```python
from build123d import *

# Parameters (mm, degrees)
F1_DEPTH     = 3.81
F2_R         = 2.032
F3_T3_ANGLE  = 90
F3_T6_ANGLE  = 90
F3_T9_DEPTH  = 16.51
F3_T12_DEPTH = 16.51


# Not quite as in the source:
# - a fillet or chamfer that OpenCascade refuses, or shapes differently, is made with other operations: its cross-section is extruded or revolved along the edge and cut away or added


with BuildPart() as f1:
    # F0 (on Top) → F1 (new body)
    with BuildSketch(Plane.XY):
        with BuildLine():
            Line((0, 36.1550717625), (0, 0))
            Line((0, 0), (50.8, 0))
            Line((50.8, 0), (50.8, 36.1550717625))
            Line((50.8, 36.1550717625), (45.72, 36.1550717625))
            Line((45.72, 36.1550717625), (45.72, 99.06))
            ThreePointArc((45.72, 99.06), (25.4, 119.38), (5.08, 99.06))
            Line((5.08, 99.06), (5.08, 36.1550717625))
            Line((5.08, 36.1550717625), (0, 36.1550717625))
        make_face()
        Polygon((21.5968196758, 48.7659722567), (5.08, 5.08), (5.08, 30.9497844428), (10.16, 30.9497844428), (10.16, 85.6342857143), (21.623824299, 55.3370357813), (18.1859140491, 55.3370357813), (18.1859140491, 48.7659722567), align=None, mode=Mode.SUBTRACT)
        Polygon((40.64, 5.08), (10.1879829027, 5.08), (25.4079982621, 45.3360045931), align=None, mode=Mode.SUBTRACT)
        Polygon((45.72, 30.9497844428), (45.72, 5.08), (29.1901726596, 48.7659722567), (32.5980894268, 48.7659722567), (32.5980894268, 55.3370357813), (29.1891943801, 55.3370357813), (40.64, 85.6237124205), (40.64, 30.9497844428), align=None, mode=Mode.SUBTRACT)
        Polygon((25.3920017379, 58.8039954069), (12.6709696314, 92.4238659741), (24.3276693245, 92.4238659741), (26.4725103977, 92.4238659741), (38.1030234, 92.4238659741), align=None, mode=Mode.SUBTRACT)
        with BuildLine():
            ThreePointArc((10.16, 99.06), (25.3630832236, 114.3000449305), (40.64, 99.1340130568))
            Line((40.64, 99.1340130568), (36.7868717318, 97.3090561919))
            Line((36.7868717318, 97.3090561919), (29.223334248, 97.3090561919))
            ThreePointArc((29.223334248, 97.3090561919), (25.4000898611, 104.8685646157), (21.5768454742, 97.3090561919))
            Line((21.5768454742, 97.3090561919), (13.8981392212, 97.3090561919))
            Line((13.8981392212, 97.3090561919), (10.16, 99.06))
        make_face(mode=Mode.SUBTRACT)
    extrude(amount=F1_DEPTH)

    # F2
    f2_edges = [f1.edges().sort_by_distance(p)[0] for p in [
        (45.72, 67.607536, 3.81),
        (50.8, 18.077536, 3.81),
        (48.26, 36.155072, 3.81),
        (2.54, 36.155072, 3.81),
        (0, 18.077536, 3.81),
    ]]
    fillet(f2_edges, radius=F2_R)

    # F3: fillet of radius 5.08 on 2 edges, made by hand


with BuildPart() as f3_tool1:
    # F3_s2 → F3_t3 (revolve)
    with BuildSketch(Plane.YZ.offset(5.08)):
        with BuildLine():
            ThreePointArc((34.1230717625, 3.81), (35.5599127419, 3.2148409794), (36.1550717625, 1.778))
            Line((36.1550717625, 1.778), (36.1550717625, 3.81))
            Line((36.1550717625, 3.81), (34.1230717625, 3.81))
        make_face()
    revolve(axis=Axis((5.08, 31.0750717625, 3.81), (0, 0, 1)), revolution_arc=F3_T3_ANGLE)


with BuildPart() as f3_tool4:
    # F3_s5 → F3_t6 (revolve)
    with BuildSketch(Plane.XZ.offset(-31.0750717625)):
        with BuildLine():
            ThreePointArc((48.768, 3.81), (50.2048409794, 3.2148409794), (50.8, 1.778))
            Line((50.8, 1.778), (50.8, 3.81))
            Line((50.8, 3.81), (48.768, 3.81))
        make_face()
    revolve(axis=Axis((45.72, 31.0750717625, 3.81), (0, 0, 1)), revolution_arc=F3_T6_ANGLE)


with BuildPart() as f3_tool7:
    # F3_s8 → F3_t9 (new body)
    with BuildSketch(Plane.XY.offset(-12.7)):
        with BuildLine():
            ThreePointArc((50.8, 31.0750717625), (49.3121024484, 34.667174211), (45.72, 36.1550717625))
            Line((45.72, 36.1550717625), (50.8, 36.1550717625))
            Line((50.8, 36.1550717625), (50.8, 31.0750717625))
        make_face()
    extrude(amount=F3_T9_DEPTH)


with BuildPart() as f3_tool10:
    # F3_s11 → F3_t12 (new body)
    with BuildSketch(Plane.XY.offset(-12.7)):
        with BuildLine():
            ThreePointArc((5.08, 36.1550717625), (1.4878975516, 34.667174211), (0, 31.0750717625))
            Line((0, 31.0750717625), (0, 36.1550717625))
            Line((0, 36.1550717625), (5.08, 36.1550717625))
        make_face()
    extrude(amount=F3_T12_DEPTH)


with BuildPart() as f1_1:
    add(f1.part)

    # F3_t13: cut F3_tool1, F3_tool4, F3_tool7, F3_tool10
    add([f3_tool1.part, f3_tool4.part, f3_tool7.part, f3_tool10.part], mode=Mode.SUBTRACT)


solid = f1_1.part
```
Model file for the job. Use its own axes, mm. A direction names the side the tool comes from. Coordinates: 2 decimals unless noted, no trailing zeros. Order: outer loops, then holes, each group sorted by start corner. A loop starts at its lowest first (then second) coordinate and runs counter-clockwise, first axis right, second up. Notation, with made-up numbers: (24.5, 79) -> (71.5, 79) arc R36 cw to (71.5, 116) -> close; hole circle Ø6 at (30, 28.5). An arc over 180 degrees is marked (long way). Return JSON: item names as keys, results as strings.
Item 1: Slice it at B-B (z = 0.95). Count the separate pieces of the cut face and the enclosed holes in it, then the cut area to 3 significant figures.
Model answer:
{"separate pieces": "1", "enclosed holes": "5", "area": "2,650 mm²"}
Item 2: Wall check: line 1 along X through (y, z) = (21, 2.75); line 2 along X through (y, z) = (104, 3.35); line 3 along X through (y, z) = (69, 3.6). Give the ranges that are in metal, low to high. Write a range as from..to.
Model answer:
{"line 1": "x = 0.25..5.08, 11.1..16.21, 34.62..39.7, 45.72..50.55", "line 2": "x = 6.46..10.98, 22.66..28.14, 39.82..44.34", "line 3": "x = 6.21..10.16, 16.45..21.53, 29.25..34.35, 40.64..44.59"}
Item 3: 3-axis set-ups, long thin cutter, end or side, ignore diameter. For faces 1 (the face through (25, 0, 2)), 2 (the face through (31.836, 75.849, 1.878)): which of +Z, -Z, +X, -X, +Y, -Y reach the whole face in a straight line?
Model answer:
{"face 1": "+Z, -Z, +X, -X, -Y", "face 2": "+Z, -Z"}
Item 4: Pin check, flat tips, straight feed: P1, Ø2, axis at x = 7, y = 26.5, coming from the +Z side; P2, Ø1.9, axis at y = 53, z = 2.5, coming from the -X side; P3, Ø1, axis at y = 53.5, z = 2, coming from the +X side. Stop position of each tip, or through.
Model answer:
{"P1": "passes through", "P2": "stops at x = 5.08", "P3": "stops at x = 45.72"}
Item 5: Mould opens along X. For faces 3 (the face through (18, 97.309, 2)), 4 (the face through (15.81, 70.7, 1.88)), 5 (the face through (5.66, 66.14, 3.2)), 6 (the face through (50.22, 15.76, 3.2)) say: pulls with the +X half, pulls with the -X half, needs draft (parallel to the pull), parting line crosses it, or undercut.
Model answer:
{"face 3": "undercut", "face 4": "undercut", "face 5": "pulls with the -X half", "face 6": "pulls with the +X half"}
Item 6: Slice it at A-A (y = 13). Write the cut outline in (x, z).
Model answer:
{"outline": "(0, 0) -> (5.08, 0) -> (5.08, 3.81) -> (2.03, 3.81) arc R2.03 ccw to (0, 1.78) -> close; (8.07, 0) -> (13.18, 0) -> (13.18, 3.81) -> (8.07, 3.81) -> close; (37.64, 0) -> (42.72, 0) -> (42.72, 3.81) -> (37.64, 3.81) -> close; (45.72, 0) -> (50.8, 0) -> (50.8, 1.78) arc R2.03 ccw to (48.77, 3.81) -> (45.72, 3.81) -> close"}
